from build123d import *

# Parameters (mm, degrees)
SKETCH1_R           = 11.5
SKETCH1_R_2         = 1.5
BOSS_EXTRUDE1_DEPTH = 10


with BuildPart() as part:
    # Sketch1 → Boss-Extrude1 (new body)
    with BuildSketch(Plane.XY):
        with BuildLine():
            Line((50, 39.5), (50, 37.5))
            ThreePointArc((50, 37.5), (50.878679656, 35.378679656), (53, 34.5))
            Line((53, 34.5), (89, 34.5))
            ThreePointArc((89, 34.5), (91.121320344, 33.621320344), (92, 31.5))
            Line((92, 31.5), (92, -22.5))
            ThreePointArc((92, -22.5), (86.142135624, -36.642135624), (72, -42.5))
            Line((72, -42.5), (-72, -42.5))
            ThreePointArc((-72, -42.5), (-86.142135624, -36.642135624), (-92, -22.5))
            Line((-92, -22.5), (-92, 31.5))
            ThreePointArc((-92, 31.5), (-91.121320344, 33.621320344), (-89, 34.5))
            Line((-89, 34.5), (-53, 34.5))
            ThreePointArc((-53, 34.5), (-50.878679656, 35.378679656), (-50, 37.5))
            Line((-50, 37.5), (-50, 39.5))
            ThreePointArc((-50, 39.5), (-49.121320344, 41.621320344), (-47, 42.5))
            Line((-47, 42.5), (47, 42.5))
            ThreePointArc((47, 42.5), (49.121320344, 41.621320344), (50, 39.5))
        make_face()
        with Locations(Location((51, -4, 0), (0, 0, 180))):
            Circle(SKETCH1_R, mode=Mode.SUBTRACT)
        with Locations((0, -39.5)):
            Circle(SKETCH1_R_2, mode=Mode.SUBTRACT)
        with Locations((84.02081528, -34.52081528)):
            Circle(SKETCH1_R_2, mode=Mode.SUBTRACT)
        with Locations((89, 31.5)):
            Circle(SKETCH1_R_2, mode=Mode.SUBTRACT)
        with Locations((47, 39.5)):
            Circle(SKETCH1_R_2, mode=Mode.SUBTRACT)
        with Locations((-47, 39.5)):
            Circle(SKETCH1_R_2, mode=Mode.SUBTRACT)
        with Locations((-89, 31.5)):
            Circle(SKETCH1_R_2, mode=Mode.SUBTRACT)
        with Locations((-84.02081528, -34.52081528)):
            Circle(SKETCH1_R_2, mode=Mode.SUBTRACT)
        with Locations((-51, -4)):
            Circle(SKETCH1_R, mode=Mode.SUBTRACT)
    extrude(amount=BOSS_EXTRUDE1_DEPTH)


solid = part.part
CAD build for the part. Positions are in the model's coordinates, mm. A direction names the side the tool comes from. Coordinates: 2 decimals unless noted, no trailing zeros. Order: outer loops, then holes, each group sorted by start corner. A loop starts at its lowest first (then second) coordinate and runs counter-clockwise, first axis right, second up.
Item 1: Drill centre lines: L1, parallel to Y at x = -89, z = 5; L2, parallel to Y at x = -47, z = 5.25; L3, parallel to X at y = -33.5, z = 7.75. Where is each one in solid material? Low to high.
Check sheet entries:
L1: y = -33.04 to 30, 33 to 34.5
L2: y = -42.5 to -14.78, 6.78 to 38, 41 to 42.5
L3: x = -88.7 to -85.12, -82.92 to 82.92, 85.12 to 88.7
Item 2: Band-saw the part on A-A on y = -4. List the corners of the cut face in (x, z).
Check sheet entries:
outline: (-92, 0) - (-62.5, 0) - (-62.5, 10) - (-92, 10) - close; (-39.5, 0) - (39.5, 0) - (39.5, 10) - (-39.5, 10) - close; (62.5, 0) - (92, 0) - (92, 10) - (62.5, 10) - close
Item 3: 3-axis set-ups, long thin cutter, end or side, ignore diameter. For faces 1 (the face through (71, 34.5, 5)), 2 (the face through (1, 1, 0)): which of +Z, -Z, +X, -X, +Y, -Y reach the whole face in a straight line?
Check sheet entries:
face 1: +Z, -Z, +X, +Y
face 2: -Z, +X, -X, +Y, -Y
Item 4: Pin check, flat tips, straight feed: pin 1 Ø18.5 at (x, y) = (-51, -4) entering from -Z; pin 2 Ø0.6 at (y, z) = (38.5, 3.5) entering from -X; pin 3 Ø1 at (y, z) = (38.5, 6.5) entering from +X; pin 4 Ø3 at (y, z) = (-30.5, 1.5) entering from +X. Stop position of each tip, or through.
Check sheet entries:
pin 1: passes through
pin 2: stops at x = -50
pin 3: stops at x = 50
pin 4: stops at x = 90.91
Item 5: Band-saw the part on B-B on x = 56. List the corners of the cut face in (y, z), plus the area to 3 significant figures.
Check sheet entries:
outline: (-42.5, 0) - (-14.36, 0) - (-14.36, 10) - (-42.5, 10) - close; (6.36, 0) - (34.5, 0) - (34.5, 10) - (6.36, 10) - close
area: 563 mm2
Item 6: Two-plate mould, pull along Y, no slides. Class faces 3 (the face through (-85.986, -36.797, 4.93)), 4 (the face through (-71, 34.5, 5)), 5 (the face through (1, 1, 10)), 6 (the face through (-62.49, -3.49, 4.93)): +Y half, -Y half, draft (parallel to the pull), parting line (faces both ways), or undercut.
Check sheet entries:
face 3: -Y half
face 4: +Y half
face 5: draft
face 6: undercut
